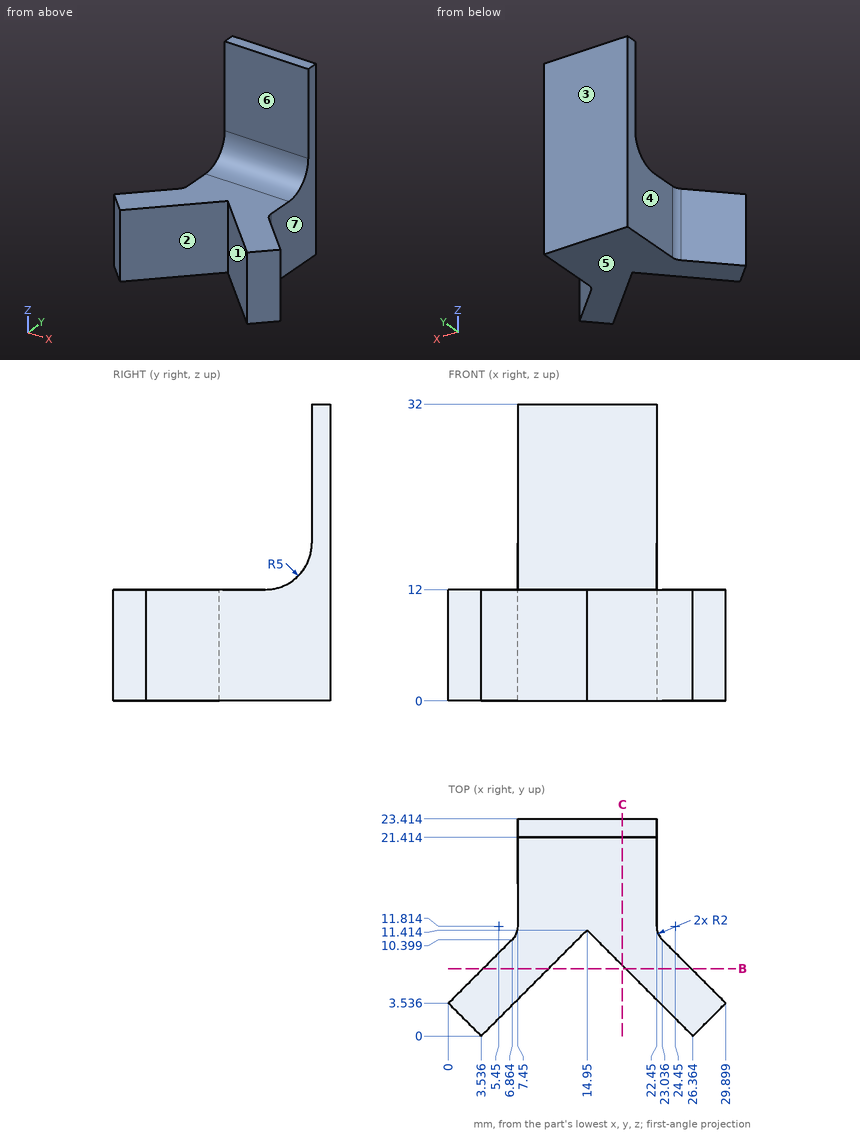
Verification items for this drawing (mm, ordinates from the low corner). A direction names the side the tool comes from. Give positions to 0.01 mm unless a question says otherwise; leave off trailing zeros. Write each loop counter-clockwise with the first axis right and the second up, starting at its lowest first coordinate (ties: lowest second). Pieces come first, ordered by that corner, then holes.
1) Gauge pin test, flat ends, axial feed: pin 1 (2 mm diameter, centred on x = 7.5, z = 5, fed in from -Y) (1 decimal); pin 2 (7.5 mm diameter, centred on x = 18, z = 26.5, fed in from -Y); pin 3 (6 mm diameter, centred on y = 16, z = 10, fed in from +X). Record the tip position at first contact, or that the pin passes through.
2) Material ranges on L1, parallel to X at y = 21.5, z = 6; L2, parallel to Z at x = 9.5, y = 13.25; L3, parallel to Y at x = 13.5, z = 28 (1 decimal), recorded low to high.
3) Section check B-B, the plane y = 7.25. Record the boundary of the cut face in (x, z) (1 decimal).
4) Section check C-C, the plane x = 18.75. Record the boundary of the cut face in (y, z) (1 decimal).
5) Access from +Z, -Z, +X, -X, +Y, -Y to the whole of each face (thin tool, end or side, straight path). Record for the marked faces 5, 6 and 7.
6) Release check for a two-part mould opening along X. For the marked faces 1, 2, 3 and 4 record: pulls with the +X half, pulls with the -X half, needs draft (parallel to the pull), parting line crosses it, or undercut.
Computed:
1. pin 1: stops at y = 3
1. pin 2: stops at y = 21.41
1. pin 3: stops at x = 22.45
2. L1: x = 7.45 to 22.45
2. L2: z = 0 to 12
2. L3: y = 21.4 to 23.4
3. outline: (3.7, 0) - (10.8, 0) - (10.8, 12) - (3.7, 12) - close; (19.1, 0) - (26.2, 0) - (26.2, 12) - (19.1, 12) - close
4. outline: (7.6, 0) - (23.4, 0) - (23.4, 32) - (21.4, 32) - (21.4, 17) arc R5 cw to (16.4, 12) - (7.6, 12) - close
5. face 5: -Z, +X, -X, +Y, -Y
5. face 6: +Z, +X, -X, -Y
5. face 7: +Z, -Z, +X, +Y
6. face 1: undercut
6. face 2: undercut
6. face 3: needs draft
6. face 4: pulls with the -X half
